from build123d import *

# Parameters (mm, degrees)
F0_R     = 31.050501
F0_R_2   = 18.320769
F1_DEPTH = 25.4
F2_T     = -2.54


with BuildPart() as f1:
    # F0 (on Front) → F1 (new body)
    with BuildSketch(Plane.XZ):
        Circle(F0_R)
        Circle(F0_R_2, mode=Mode.SUBTRACT)
    extrude(amount=F1_DEPTH)

    # F2
    f2_openings = [f1.faces().sort_by_distance(p)[0] for p in [
        (-30.17226, -25.4, 0),
    ]]
    offset(amount=F2_T, openings=f2_openings)


solid = f1.part
Geometry check sheet. Reference: the model listing, model coordinates, mm. A direction names the side the tool comes from. Round coordinates to 2 decimals unless told otherwise and drop trailing zeros. Order: outer loops, then holes, each group sorted by start corner. A loop starts at its lowest first (then second) coordinate and runs counter-clockwise, first axis right, second up. Notation, with made-up numbers: M 33.25,23.25 L 75.25,23.25 A19 ccw 75.25,56.25 Z; hole C 36,2.25 d5. An arc over 180 degrees is marked long. Write each question's results on one line, items separated by ' | '. Start each with the question number.
1. Go/stop test with flat-tipped pins: P1, Ø1, axis at y = -16.5, z = -6.5, coming from the +X side; P2, Ø6, axis at x = 6.5, z = 11.5, coming from the +Y side; P3, Ø4, axis at y = -11.5, z = -14, coming from the -X side; P4, Ø6, axis at y = -4.5, z = 15.5, coming from the -X side. Record where each tip stops, or that it passes through.
2. Material ranges on L1, parallel to Z at x = 0, y = -8; L2, parallel to Z at x = 3, y = -11.75; L3, parallel to X at y = -21.25, z = -14, recorded low to high. Write a range as from..to.
3. Cross-section at C-C on y = -14.25. Record the boundary of the cut face in (x, z), plus the area to 3 significant figures.
4. Cross-section at D-D on z = -24.5. Record the boundary of the cut face in (x, y), plus the area to 3 significant figures.
5. Cross-section at A-A on x = 0. Record the boundary of the cut face in (y, z).
6. Set-up check for faces 4 (the face through (-22.625, -13.81, -17.348)), 5 (the face through (16.924, -12.522, -7.017)): record each of +Z, -Z, +X, -X, +Y, -Y from which the full face is reachable in a straight line by a thin tool's end or side.
7. Cross-section at B-B on z = 14.5. Record the boundary of the cut face in (x, y), plus the area to 3 significant figures.
8. Draft check along Z on faces 1 (the face through (-4.042, -12.522, 30.786)), 2 (the face through (1.45, -25.4, -18.45)), 3 (the face through (-4.522, -13.81, -20.365)). Enter one of: pulls with the +Z half, pulls with the -Z half, needs draft (parallel to the pull), parting line crosses it, or undercut.
Resolved:
1) P1: x = 30.47 | P2: through | P3: x = -28.64 | P4: x = -28.42
2) L1: -31.05..-28.51, -20.86..-18.32, 18.32..20.86, 28.51..31.05 | L2: -30.91..-28.35, -20.64..-18.07, 18.07..20.64, 28.35..30.91 | L3: -27.72..-24.84, -15.47..-11.82, 11.82..15.47, 24.84..27.72
3) outline: C 0,0 d62.1; C 0,0 d41.72; hole C 0,0 d57.02; hole C 0,0 d36.64 | area: 788 mm2
4) outline: M -19.08,-25.4 L -14.58,-25.4 L -14.58,-2.54 L 14.58,-2.54 L 14.58,-25.4 L 19.08,-25.4 L 19.08,0 L -19.08,0 Z | area: 302 mm2
5) outline: M -25.4,-31.05 L 0,-31.05 L 0,-18.32 L -25.4,-18.32 L -25.4,-20.86 L -2.54,-20.86 L -2.54,-28.51 L -25.4,-28.51 Z; M -25.4,18.32 L 0,18.32 L 0,31.05 L -25.4,31.05 L -25.4,28.51 L -2.54,28.51 L -2.54,20.86 L -25.4,20.86 Z
6) face 4: -Y | face 5: +Y, -Y
7) outline: M -27.46,-25.4 L -24.55,-25.4 L -24.55,-2.54 L -15,-2.54 L -15,-25.4 L -11.2,-25.4 L -11.2,0 L -27.46,0 Z; M 11.2,-25.4 L 15,-25.4 L 15,-2.54 L 24.55,-2.54 L 24.55,-25.4 L 27.46,-25.4 L 27.46,0 L 11.2,0 Z | area: 389 mm2
8) face 1: parting line crosses it | face 2: needs draft | face 3: undercut
